```python
from build123d import *

# Parameters (mm, degrees)
SKETCH_1_R      = 1.7
EXTRUDE_1_DEPTH = 2


with BuildPart() as part:
    # 草图1 → 凸台-拉伸1 (new body)
    with BuildSketch(Plane.XY):
        Polygon((0, 0), (40, 0), (40, 15), (15, 15), (15, 40), (0, 40), align=None)
        with Locations((20, 7.5)):
            Circle(SKETCH_1_R, mode=Mode.SUBTRACT)
        with Locations((34, 7.5)):
            Circle(SKETCH_1_R, mode=Mode.SUBTRACT)
        with Locations(Location((7.5, 34, 0), (0, 0, 180))):
            Circle(SKETCH_1_R, mode=Mode.SUBTRACT)
        with Locations(Location((7.5, 20, 0), (0, 0, 180))):
            Circle(SKETCH_1_R, mode=Mode.SUBTRACT)
    extrude(amount=EXTRUDE_1_DEPTH)


solid = part.part
```
For this review, take the finished solid that the model builds, in its own axes (mm). Round coordinates to 2 decimals unless told otherwise and drop trailing zeros. Write each loop counter-clockwise with the first axis right and the second up, starting at its lowest first coordinate (ties: lowest second). Pieces come first, ordered by that corner, then holes. Notation, with made-up numbers: (83, 83.25) - (138, 83.25) arc R16 ccw to (138, 114.25) - close; hole circle Ø3 at (59, 50.25). An arc over 180 degrees is marked (long way). Answer as a JSON object with one key per item and string values.
1. We need section A-A on y = 34. Give the boundary of the cut face in (x, z).
Response values:
{"outline": "(0, 0) - (5.8, 0) - (5.8, 2) - (0, 2) - close; (9.2, 0) - (15, 0) - (15, 2) - (9.2, 2) - close"}
2. To check wall thickness, follow line 1 along Y through (x, z) = (7.5, 0.95); line 2 along Y through (x, z) = (20, 1.55). State the ranges of each line that lie inside material, in increasing order.
Response values:
{"line 1": "y = 0 to 18.3, 21.7 to 32.3, 35.7 to 40", "line 2": "y = 0 to 5.8, 9.2 to 15"}
3. We need section B-B on z = 0.55. Give the boundary of the cut face in (x, y), then the cut area to 3 significant figures.
Response values:
{"outline": "(0, 0) - (40, 0) - (40, 15) - (15, 15) - (15, 40) - (0, 40) - close; hole circle Ø3.4 at (7.5, 20); hole circle Ø3.4 at (7.5, 34); hole circle Ø3.4 at (20, 7.5); hole circle Ø3.4 at (34, 7.5)", "area": "939 mm2"}
4. For pin 1 Ø10 at (x, y) = (19, 26) entering from +Z; pin 2 Ø0.6 at (x, z) = (27.5, 0.5) entering from +Y, all flat-tipped, find the tip position at first contact; note any pin that passes through.
Response values:
{"pin 1": "stops at z = 2", "pin 2": "stops at y = 15"}
5. We need section C-C on x = 7.5. Give the boundary of the cut face in (y, z), then the cut area to 3 significant figures.
Response values:
{"outline": "(0, 0) - (18.3, 0) - (18.3, 2) - (0, 2) - close; (21.7, 0) - (32.3, 0) - (32.3, 2) - (21.7, 2) - close; (35.7, 0) - (40, 0) - (40, 2) - (35.7, 2) - close", "area": "66.4 mm2"}
6. Draft analysis for pull direction Y (two halves, no side actions). For faces 1 (the face through (15, 27, 1)), 2 (the face through (7.721, 18.314, 0.986)), 3 (the face through (28, 15, 1)), state which applies: +Y half, -Y half, draft (parallel to the pull), parting line (faces both ways), or undercut.
Response values:
{"face 1": "draft", "face 2": "undercut", "face 3": "+Y half"}
